Autodesk Inventor part; units mm, degrees
ref_plane "YZ Plane" through (0, 0, 0) normal (1, 0, 0) x (0, 1, 0)
ref_plane "XZ Plane" through (0, 0, 0) normal (0, 1, 0) x (-1, 0, 0)
ref_plane "XY Plane" through (0, 0, 0) normal (0, 0, 1) x (1, 0, 0)
sketch "Sketch1" plane through (0, 0, 0) normal (0, 0, 1) x (1, 0, 0)
  line L0 (-30.1, -12.5) -> (30.1, -12.5)
  line L1 (38.1, -4.5) -> (38.1, 4.5)
  line L2 (30.1, 12.5) -> (-30.1, 12.5)
  line L3 (-38.1, 4.5) -> (-38.1, -4.5)
  line L4 (-38.1, -12.5) -> (38.1, 12.5) construction
  line L5 (38.1, -12.5) -> (-38.1, 12.5) construction
  line L6 (-38.1, 0) -> (38.1, 0) construction
  line L7 (0, 12.5) -> (0, -12.5) construction
  circle A0 centre (0, 0) radius 25.4 construction
  line L8 (-19.05, 12.5) -> (19.05, 12.5) construction
  line L9 (19.05, 12.5) -> (19.05, -12.5)
  line L10 (19.05, -12.5) -> (-19.05, -12.5) construction
  line L11 (-19.05, -12.5) -> (-19.05, 12.5)
  line L12 (-19.05, 12.5) -> (19.05, -12.5) construction
  line L13 (19.05, 12.5) -> (-19.05, -12.5) construction
  circle A1 centre (-25.4, 0) radius 2.3
  circle A2 centre (25.4, 0) radius 2.3
  arc A3 (-30.1, 12.5) -> (-38.1, 4.5) centre (-30.1, 4.5) ccw
  arc A4 (-38.1, -4.5) -> (-30.1, -12.5) centre (-30.1, -4.5) ccw
  arc A5 (30.1, -12.5) -> (38.1, -4.5) centre (30.1, -4.5) ccw
  arc A6 (38.1, 4.5) -> (30.1, 12.5) centre (30.1, 4.5) ccw
  dimension "d2" = 50.8
  dimension "d0" = 76.2
  dimension "d1" = 25
  dimension "d3" = 38.1
  dimension "d4" = 25
  dimension "d5" = 4.6
  dimension "d6" = 8
extrude "Extrusion1" add sketch "Sketch1" against normal blind 3
extrude "Extrusion2" add sketch "Sketch1" along normal blind 44.45 contours L11 L2 L9 L0
sketch "Sketch2" plane through (19.05, -12.5, 0) normal (1, 0, 0) x (0, 0, -1)
  line L0 (-44.45, 0) -> (-44.45, 25) construction
  line L1 (-44.45, 12.5) -> (3, 12.5) construction
  line L2 (3, 8) -> (3, 17) construction
  circle A0 centre (-37.45, 12.5) radius 3
  point P0 (0, 12.5)
  dimension "d11" = 6
  dimension "d12" = 7
extrude "Extrusion3" cut sketch "Sketch2" against normal blind 44.45
fillet "Fillet1" radius 1 4 edges at (19.05, -12.5, 22.225) (19.05, 12.5, 22.225) (-19.05, 12.5, 22.225) (-19.05, -12.5, 22.225)
fillet "Fillet2" radius 1 8 edges at (-18.7571, -12.2071, 44.45) (0, -12.5, 44.45) (18.7571, -12.2071, 44.45) (19.05, 0, 44.45) (18.7571, 12.2071, 44.45) (0, 12.5, 44.45) (-18.7571, 12.2071, 44.45) (-19.05, 0, 44.45)
fillet "Fillet3" radius 0.5 14 edges at (-35.7569, -10.1569, 0) (-18.55, -12.5, 0) (-24.575, -12.5, 0) (-35.7569, 10.1569, 0) (-18.55, 12.5, 0) (-24.575, 12.5, 0) (-38.1, 0, 0) (38.1, 0, 0) (35.7569, 10.1569, 0) (18.55, 12.5, 0) (24.575, 12.5, 0) (18.55, -12.5, 0) (24.575, -12.5, 0) (35.7569, -10.1569, 0)
properties part number "camstand1.75inch tall"
Input: part model. Units: mm. Frame: model coordinates. A direction names the side the tool comes from. Coordinates: 2 decimals unless noted, no trailing zeros. Write each loop counter-clockwise with the first axis right and the second up, starting at its lowest first coordinate (ties: lowest second). Pieces come first, ordered by that corner, then holes. Notation, with made-up numbers: M 56,62.5 L 79,62.5 A25 ccw 79,77.5 Z; hole C 72,30 d2. An arc over 180 degrees is marked long. Answer as a JSON object with one key per item and string values. Group by question number.
(1) Contact query for flat-ended pins moving along their axis: P1, Ø7.5, axis at x = -25.4, y = 0, coming from the +Z side; P2, Ø6, axis at y = 4.5, z = 9.5, coming from the +X side; P3, Ø3, axis at y = 0.5, z = 21, coming from the -X side. Output: stop coordinate, or through.
(2) Mould query, pull axis Y, two halves, no side actions, for faces 1 (the face through (0.27, 0.9, 34.59)), 2 (the face through (-1, 0, -3)), 3 (the face through (-35.694, 10.219, -1.732)). Classes: pulls with the +Y half, pulls with the -Y half, needs draft (parallel to the pull), parting line crosses it, or undercut.
(3) Section D-D on y = 0. Output: boundary loops of the cut face in (x, z), plus the area to 3 significant figures.
(4) Ray query, line 1 along Y through (x, z) = (25.4, -1.1); line 2 along Y through (x, z) = (6.5, 37.45); line 3 along X through (y, z) = (-1.5, 11). Return the intervals inside material, ascending. Write a range as [from, to].
(5) Section C-C on x = -11. Output: boundary loops of the cut face in (y, z), plus the area to 3 significant figures.
(6) Set-up query: faces 4 (the face through (0, 0, 44.45)), 5 (the face through (-19.05, 0, 21)), 6 (the face through (28, 0, 0)). Return all of +Z, -Z, +X, -X, +Y, -Y with unobstructed straight access to the full face (end or side cutting, diameter ignored); none if empty.
(7) Section A-A on z = 37.45. Output: boundary loops of the cut face in (x, y).
(8) Section B-B on x = -25.4. Output: boundary loops of the cut face in (y, z).
Result set:
{
 "1": {"P1": "stops at z = 0", "P2": "stops at x = 19.05", "P3": "stops at x = -19.05"},
 "2": {"face 1": "undercut", "face 2": "needs draft", "face 3": "pulls with the +Y half"},
 "3": {"outline": "M -38.1,-3 L -27.7,-3 L -27.7,0 L -37.6,0 A0.5 ccw -38.1,-0.5 Z; M -23.1,-3 L 23.1,-3 L 23.1,0 L 19.05,0 L 19.05,34.45 L -19.05,34.45 L -19.05,0 L -23.1,0 Z; M -19.05,40.45 L 19.05,40.45 L 19.05,43.45 A1 ccw 18.05,44.45 L -18.05,44.45 A1 ccw -19.05,43.45 Z; M 27.7,-3 L 38.1,-3 L 38.1,-0.5 A0.5 ccw 37.6,0 L 27.7,0 Z", "area": "1,670 mm2"},
 "4": {"line 1": "y = [-12.5, -2.3], [2.3, 12.5]", "line 2": "y = [-12.5, -3], [3, 12.5]", "line 3": "x = [-19.05, 19.05]"},
 "5": {"outline": "M -12.5,-3 L 12.5,-3 L 12.5,43.45 A1 ccw 11.5,44.45 L -11.5,44.45 A1 ccw -12.5,43.45 Z; hole C 0,37.45 d6", "area": "1,160 mm2"},
 "6": {"face 4": "+Z, +X, -X, +Y, -Y", "face 5": "+Z, -X, +Y, -Y", "face 6": "+Z, +X, +Y, -Y"},
 "7": {"outline": "M -19.05,-11.5 A1 ccw -18.05,-12.5 L 18.05,-12.5 A1 ccw 19.05,-11.5 L 19.05,-3 L -19.05,-3 Z; M -19.05,3 L 19.05,3 L 19.05,11.5 A1 ccw 18.05,12.5 L -18.05,12.5 A1 ccw -19.05,11.5 Z"},
 "8": {"outline": "M -12.5,-3 L -2.3,-3 L -2.3,0 L -12,0 A0.5 ccw -12.5,-0.5 Z; M 2.3,-3 L 12.5,-3 L 12.5,-0.5 A0.5 ccw 12,0 L 2.3,0 Z"}
}
